Can you work these out from the model? Positions are in its coordinate system, mm. Give positions to 0.01 mm unless a question says otherwise; leave off trailing zeros. Order: outer loops, then holes, each group sorted by start corner. A loop starts at its lowest first (then second) coordinate and runs counter-clockwise, first axis right, second up. Notation, with made-up numbers: M 13.5,61 L 47.5,61 A18 ccw 47.5,74 Z; hole C 56,26.5 d5. An arc over 180 degrees is marked long. One line per question, with ' | ' between items. Start each with the question number.
1) If we section it at B-B, the plane x = 0: Please give me the cut outline in (y, z) (3 decimals), plus the area to 3 significant figures.
2) If we section it at D-D, the plane x = -11: Please give me the cut outline in (y, z) (3 decimals).
3) If we section it at C-C, the plane z = -1.5: State how many separate pieces and enclosed holes the cut face has, plus the area to 3 significant figures.
4) If we section it at A-A, the plane y = 0: Please give me the cut outline in (x, z) (3 decimals), plus the area to 3 significant figures.
5) Thinking about a two-plate mould opening in Y: for faces 1 (the cylindrical face through (-23.49, -20.414, -1.61)), 2 (the cylindrical face through (16.613, 17.465, -2.917)), 3 (the flat face through (-12, 10, 0)), which applies, +Y half, -Y half, draft (parallel to the pull), parting line (faces both ways), or undercut?
6) Please list where these lines run through material, in increasing order: line 1 along Y through (x, z) = (0, -1.3) (3 decimals); line 2 along Y through (x, z) = (19.05, -2.8) (3 decimals); line 3 along X through (y, z) = (-9, -2.2). Write a range as [from, to].
7) I'm going to push a flat-ended pin straight in: pin 1 Ø6 at (x, y) = (9.5, -3.5) entering from -Z. Where does the tip first touch, or does it pass through?
Autodesk Inventor part; units mm, degrees
ref_plane "YZ Plane" through (0, 0, 0) normal (1, 0, 0) x (0, 1, 0)
ref_plane "XZ Plane" through (0, 0, 0) normal (0, 1, 0) x (-1, 0, 0)
ref_plane "XY Plane" through (0, 0, 0) normal (0, 0, 1) x (1, 0, 0)
sketch "Sketch1" plane through (0, 0, 0) normal (0, 0, 1) x (1, 0, 0)
  line L0 (-31.75, 22.225) -> (31.75, 22.225)
  line L1 (31.75, 22.225) -> (31.75, -22.225)
  line L2 (31.75, -22.225) -> (-31.75, -22.225)
  line L3 (-31.75, -22.225) -> (-31.75, 22.225)
  circle A0 centre (0, 0) radius 13.716
  circle A1 centre (0, 0) radius 13.6017
  circle A2 centre (13.7482, -7.9375) radius 1.6193
  circle A3 centre (0, 0) radius 15.875 construction
  circle A4 centre (0, 15.875) radius 1.6193
  circle A5 centre (-13.7482, -7.9375) radius 1.6193
  circle A6 centre (0, 0) radius 21.59 construction
  line L4 (0, 0) -> (13.7482, -7.9375)
  line L5 (0, 0) -> (0, -22.225)
  line L6 (0, 0) -> (0, -22.225)
  line L7 (-31.75, 22.225) -> (-25.4, 22.225)
  line L8 (-25.4, 22.225) -> (-25.4, -22.225)
  line L9 (-25.4, -22.225) -> (-31.75, -22.225)
  line L10 (-31.75, -22.225) -> (-31.75, 22.225)
  line L11 (31.75, 22.225) -> (25.4, 22.225)
  line L12 (25.4, 22.225) -> (25.4, -22.225)
  line L13 (25.4, -22.225) -> (31.75, -22.225)
  line L14 (31.75, -22.225) -> (31.75, 22.225)
  point P0 (-19.05, 17.145)
  point P1 (-19.05, -17.145)
  point P2 (19.05, -17.145)
  point P3 (19.05, 17.145)
  dimension "d0" = 44.45
  dimension "d1" = 63.5
  dimension "d2" = 31.75
  dimension "d3" = 22.225
  dimension "d4" = 27.432
  dimension "d7" = 3.2385
  dimension "d9" = 15.875
  dimension "d15" = 360
  dimension "d17" = 43.18
  dimension "d18" = 5.08
  dimension "d19" = 5.08
  dimension "d20" = 19.05
  dimension "d21" = 19.05
  dimension "d31" = 34.29
  dimension "d32" = 38.1
  dimension "d35" = 60
  dimension "d36" = 6.35
  dimension "d37" = 6.35
extrude "Extrusion1" add sketch "Sketch1" against normal blind 3.175
hole "Hole1" at (-19.05, 17.145, 0) at (-19.05, -17.145, 0) at (19.05, -17.145, 0) at (19.05, 17.145, 0) direction (0, 0, -1) diameter 4.9149 end through all countersink diameter 9.525 countersink angle 82
extrude "Extrusion2" cut sketch "Sketch1" against normal through all contours L0 L8 L2 L3 | L0 L1 L2 L12
fillet "Fillet1" radius 6.35 4 edges at (25.4, 22.225, -1.5875) (25.4, -22.225, -1.5875) (-25.4, -22.225, -1.5875) (-25.4, 22.225, -1.5875)
properties part number "Dewalt Drill Cap Rotation plate"
Results found:
1) outline: M -22.225,-3.175 L -13.716,-3.175 L -13.716,0 L -22.225,0 Z; M 13.716,-3.175 L 14.256,-3.175 L 14.256,0 L 13.716,0 Z; M 17.494,-3.175 L 22.225,-3.175 L 22.225,0 L 17.494,0 Z | area: 43.7 mm²
2) outline: M -22.225,-3.175 L -8.193,-3.175 L -8.193,0 L -22.225,0 Z; M 8.193,-3.175 L 22.225,-3.175 L 22.225,0 L 8.193,0 Z
3) separate pieces: 1 | enclosed holes: 8 | area: 1,460 mm²
4) outline: M -25.4,-3.175 L -13.716,-3.175 L -13.716,0 L -25.4,0 Z; M 13.716,-3.175 L 25.4,-3.175 L 25.4,0 L 13.716,0 Z | area: 74.2 mm²
5) face 1: -Y half | face 2: undercut | face 3: draft
6) line 1: y = [-22.225, -13.716], [13.716, 14.256], [17.494, 22.225] | line 2: y = [-22.225, -19.602], [-14.688, 14.688], [19.602, 22.225] | line 3: x = [-25.4, -14.97], [-12.53, -10.35], [10.35, 12.53], [14.97, 25.4]
7) pin 1: passes through
